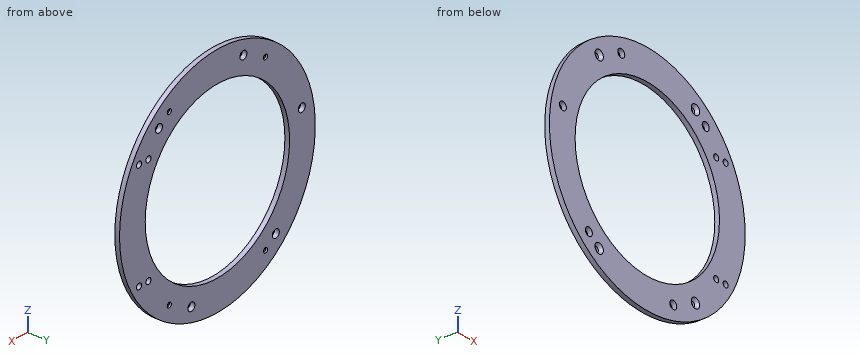
```python
from build123d import *

# Parameters (mm, degrees)
GEMINI_SKIRT_F_2_R                            = 77.4954
GEMINI_SKIRT_F_2_R_2                          = 57.15
GEMINI_SKIRT_F_DEPTH                          = 3.175
M5_CLEARANCE_HOLE1_D                          = 5.5
M5_CLEARANCE_HOLE1_DEPTH                      = 3.175
CSK_FOR_4_FLAT_HEAD_MACHINE_SCREW1_AT_2_COUNT = 2
CSK_FOR_4_FLAT_HEAD_MACHINE_SCREW1_AT_2_PITCH = 76.2
CSK_FOR_4_FLAT_HEAD_MACHINE_SCREW1_AT_3_COUNT = 2
CSK_FOR_4_FLAT_HEAD_MACHINE_SCREW1_AT_3_PITCH = 113.740110937
CSK_FOR_4_FLAT_HEAD_MACHINE_SCREW1_AT_4_COUNT = 2
CSK_FOR_4_FLAT_HEAD_MACHINE_SCREW1_AT_4_PITCH = 136.906
F_5_32_0_15625_DIAMETER_HOLE1_D               = 3.96875
F_5_32_0_15625_DIAMETER_HOLE1_DEPTH           = 3.175


with BuildPart() as part:
    # GEMINI_SKIRT-F 2 → GEMINI_SKIRT_F (new body)
    with BuildSketch(Plane(origin=(0, -40.33266, 0), x_dir=(1, 0, 0), z_dir=(0, 1, 0))):
        Circle(GEMINI_SKIRT_F_2_R)
        Circle(GEMINI_SKIRT_F_2_R_2, mode=Mode.SUBTRACT)
    extrude(amount=-GEMINI_SKIRT_F_DEPTH)

    # M5 Clearance Hole1
    with Locations(Plane(origin=(0, -40.33266, 0), x_dir=(1, 0, 0), z_dir=(0, 1, 0))):
        with Locations((20.584214093, 65.28478643), (46.246176482, -50.468845537), (-20.584214093, -65.28478643), (-46.246176482, 50.468845537), (-66.830390575, -14.815940893)):
            Hole(M5_CLEARANCE_HOLE1_D / 2, depth=M5_CLEARANCE_HOLE1_DEPTH)

    # Sketch8 → CSK for #4 Flat Head Machine Screw1 (revolve, cut)
    with BuildSketch(Plane(origin=(38.1, -43.50766, -56.870055469), x_dir=(0, 0, -1), z_dir=(1, 0, 0))):
        Polygon((0, 0), (0, 3.175), (1.63195, 3.175), (1.63195, 1.921172758), (3.302, 0), align=None)
    csk_for_4_flat_head_machine_screw1 = revolve(axis=Axis((38.1, -49.85766, -56.870055469), (0, 1, 0)), mode=Mode.SUBTRACT)

    # CSK for #4 Flat Head Machine Screw1 at 2: CSK for #4 Flat Head Machine Screw1 ×2
    with Locations(*[(-i * CSK_FOR_4_FLAT_HEAD_MACHINE_SCREW1_AT_2_PITCH, 0, 0) for i in range(1, CSK_FOR_4_FLAT_HEAD_MACHINE_SCREW1_AT_2_COUNT)]):
        add(csk_for_4_flat_head_machine_screw1, mode=Mode.SUBTRACT)

    # CSK for #4 Flat Head Machine Screw1 at 3: CSK for #4 Flat Head Machine Screw1 ×2
    with Locations(*[(0, 0, i * CSK_FOR_4_FLAT_HEAD_MACHINE_SCREW1_AT_3_PITCH) for i in range(1, CSK_FOR_4_FLAT_HEAD_MACHINE_SCREW1_AT_3_COUNT)]):
        add(csk_for_4_flat_head_machine_screw1, mode=Mode.SUBTRACT)

    # CSK for #4 Flat Head Machine Screw1 at 4: CSK for #4 Flat Head Machine Screw1 ×2
    with Locations(*[Vector(-0.556586271, 0, 0.830789819) * (i * CSK_FOR_4_FLAT_HEAD_MACHINE_SCREW1_AT_4_PITCH) for i in range(1, CSK_FOR_4_FLAT_HEAD_MACHINE_SCREW1_AT_4_COUNT)]):
        add(csk_for_4_flat_head_machine_screw1, mode=Mode.SUBTRACT)

    # 5/32 (0.15625) Diameter Hole1
    with Locations(Plane(origin=(0, -40.33266, 0), x_dir=(1, 0, 0), z_dir=(0, 1, 0))):
        with Locations((62.031667622, -35.814), (54.576319847, -35.814), (54.576319847, 35.814), (62.031667622, 35.814)):
            Hole(F_5_32_0_15625_DIAMETER_HOLE1_D / 2, depth=F_5_32_0_15625_DIAMETER_HOLE1_DEPTH)


solid = part.part
```
Work out the finished part from the listing and answer in its coordinate system (mm). Coordinates: 2 decimals unless noted, no trailing zeros. Loops run counter-clockwise (first coordinate to the right, second up) from the corner with the lowest first, then second, coordinate; pieces in that order, holes last.
1) Section C-C (y = -42.65) is taken. Give the number of separate pieces and of enclosed holes in the cut face, plus the area to 3 significant figures.
Results:
separate pieces: 1
enclosed holes: 14
area: 8,360 mm2
2) Section A-A (z = 0) is taken. Give the vertices of the cut face in (x, y), plus the area to 3 significant figures.
Results:
outline: (-77.5, -43.51) - (-57.15, -43.51) - (-57.15, -40.33) - (-77.5, -40.33) - close; (57.15, -43.51) - (77.5, -43.51) - (77.5, -40.33) - (57.15, -40.33) - close
area: 129 mm2
3) A flat-ended cylindrical pin translates along its axis: pin 1 (5 mm diameter, centred on x = -38.1, z = 56.87, fed in from -Y). Find the tip coordinate at first contact, or state that the pin passes through.
Results:
pin 1: stops at y = -42.59
4) Section B-B (x = 0) is taken. Give the vertices of the cut face in (y, z).
Results:
outline: (-43.51, -77.5) - (-40.33, -77.5) - (-40.33, -57.15) - (-43.51, -57.15) - close; (-43.51, 57.15) - (-40.33, 57.15) - (-40.33, 77.5) - (-43.51, 77.5) - close
5) Consider probe 1 along X at (y, z) = (-42.2, 16); probe 2 along X at (y, z) = (-40.8, 2) (3 decimals); probe 3 along Z at (x, y) = (38.1, -40.6). Determine where each line is inside the solid, lowest interval first.
Results:
probe 1: x = -75.83 to -69.31, -64.35 to -54.86, 54.86 to 75.83
probe 2: x = -77.47 to -57.115, 57.115 to 77.47
probe 3: z = -67.48 to -58.5, -55.24 to -42.6, 42.6 to 55.24, 58.5 to 67.48
